```python
from build123d import *

# Parameters (mm, degrees)
EXTRUDE_1_DEPTH          = 10
SKETCH_2_R               = 16
CUT_EXTRUDE_1_DEPTH      = 10
SKETCH_3_R               = 5
CUT_EXTRUDE_2_DEPTH      = 10
SKETCH_6_R               = 2
CUT_EXTRUDE_4_DEPTH      = 10
PATTERN_CIRCULAR_1_COUNT = 4


with BuildPart() as part:
    # 草图1 → 凸台-拉伸1 (new body)
    with BuildSketch(Plane.XY):
        Polygon((50, -85), (-50, -85), (-50, -40), (-50, 85), (50, 85), (50, 0), align=None)
    extrude(amount=EXTRUDE_1_DEPTH)

    # 草图2 → 切除-拉伸1 (cut)
    with BuildSketch(Plane.XY.offset(10)):
        Circle(SKETCH_2_R)
    extrude(amount=-CUT_EXTRUDE_1_DEPTH, mode=Mode.SUBTRACT)

    # 草图3 → 切除-拉伸2 (cut)
    with BuildSketch(Plane.XY.offset(10)):
        with Locations((0, -72)):
            Circle(SKETCH_3_R)
        with Locations((35, -72)):
            Circle(SKETCH_3_R)
        with Locations((-35, -72)):
            Circle(SKETCH_3_R)
    cut_extrude_2 = extrude(amount=-CUT_EXTRUDE_2_DEPTH, mode=Mode.SUBTRACT)

    # 草图6 → 切除-拉伸4 (cut)
    with BuildSketch(Plane.XY.offset(10)):
        with Locations((0, 21)):
            Circle(SKETCH_6_R)
    cut_extrude_4 = extrude(amount=-CUT_EXTRUDE_4_DEPTH, mode=Mode.SUBTRACT)

    # 阵列(圆周)1: 切除-拉伸4 ×4 about axis
    pattern_circular_1_axis = Axis((0, 0, 0), (0, 0, 1))
    for i in range(1, PATTERN_CIRCULAR_1_COUNT):
        add(cut_extrude_4.rotate(pattern_circular_1_axis, i * 360 / PATTERN_CIRCULAR_1_COUNT), mode=Mode.SUBTRACT)

    # 镜向1: 切除-拉伸2 across plane
    add(cut_extrude_2.mirror(Plane.ZX), mode=Mode.SUBTRACT)


solid = part.part
```
Design review of the part built by this model. Coordinates are the model's own, in mm. Give positions to 0.01 mm unless a question says otherwise; leave off trailing zeros. Order: outer loops, then holes, each group sorted by start corner. A loop starts at its lowest first (then second) coordinate and runs counter-clockwise, first axis right, second up. Notation, with made-up numbers: (40.25, 23) - (93.25, 23) arc R38 ccw to (93.25, 61) - close; hole circle Ø5 at (-3, 61.25). An arc over 180 degrees is marked (long way). Use a Markdown table: item, result. Add a question column.
(1) Add section A-A on x = 21. Give the boundary of the cut face in (y, z), then the cut area to 3 significant figures.
(2) Add section D-D on x = 0. Give the boundary of the cut face in (y, z), then the cut area to 3 significant figures.
(3) Add section B-B on y = 21. Give the boundary of the cut face in (x, z).
(4) Wall thickness on probe 1 along Y at (x, z) = (35, 6); probe 2 along X at (y, z) = (72, 4.25); probe 3 along Y at (x, z) = (-3, 5): over which ranges is each line inside the solid? List them lowest first. Write a range as [from, to].
(5) Add section C-C on y = -72. Give the boundary of the cut face in (x, z).
(6) Mouldability with a two-part tool opening along Y and no side actions: class faces 1 (the face through (1, -85, 5)), 2 (the face through (-50, 1, 5)), 3 (the face through (3, -68, 5)) as +Y half, -Y half, draft (parallel to the pull), parting line (faces both ways), or undercut.
Report:
| question | item | result |
|---|---|---|
| 1 | outline | (-85, 0) - (-2, 0) - (-2, 10) - (-85, 10) - close; (2, 0) - (85, 0) - (85, 10) - (2, 10) - close |
| 1 | area | 1,660 mm² |
| 2 | outline | (-85, 0) - (-77, 0) - (-77, 10) - (-85, 10) - close; (-67, 0) - (-23, 0) - (-23, 10) - (-67, 10) - close; (-19, 0) - (-16, 0) - (-16, 10) - (-19, 10) - close; (16, 0) - (19, 0) - (19, 10) - (16, 10) - close; (23, 0) - (67, 0) - (67, 10) - (23, 10) - close; (77, 0) - (85, 0) - (85, 10) - (77, 10) - close |
| 2 | area | 1,100 mm² |
| 3 | outline | (-50, 0) - (-2, 0) - (-2, 10) - (-50, 10) - close; (2, 0) - (50, 0) - (50, 10) - (2, 10) - close |
| 4 | probe 1 | y = [-85, -77], [-67, 67], [77, 85] |
| 4 | probe 2 | x = [-50, -40], [-30, -5], [5, 30], [40, 50] |
| 4 | probe 3 | y = [-85, -76], [-68, -15.72], [15.72, 68], [76, 85] |
| 5 | outline | (-50, 0) - (-40, 0) - (-40, 10) - (-50, 10) - close; (-30, 0) - (-5, 0) - (-5, 10) - (-30, 10) - close; (5, 0) - (30, 0) - (30, 10) - (5, 10) - close; (40, 0) - (50, 0) - (50, 10) - (40, 10) - close |
| 6 | face 1 | -Y half |
| 6 | face 2 | draft |
| 6 | face 3 | undercut |
